from build123d import *

# Parameters (mm, degrees)
SKETCH1_W           = 150
SKETCH1_H           = 150
BOSS_EXTRUDE1_DEPTH = 1.5
CUT_EXTRUDE1_DEPTH  = 3
SKETCH3_R           = 1.55
CUT_EXTRUDE2_DEPTH  = 3
SKETCH6_R           = 1.3
SKETCH6_R_2         = 2.55
CUT_EXTRUDE9_DEPTH  = 3
SKETCH7_W           = 20
SKETCH7_H           = 50
SKETCH7_W_2         = 48
SKETCH7_H_2         = 40
SKETCH7_W_3         = 74
SKETCH7_H_3         = 46
CUT_EXTRUDE10_DEPTH = 3
FILLET1_R           = 4


with BuildPart() as part:
    # Sketch1 → Boss-Extrude1 (new body, symmetric)
    with BuildSketch(Plane(origin=(0, 0, 0), x_dir=(1, 0, 0), z_dir=(0, 1, 0))):
        Rectangle(SKETCH1_W, SKETCH1_H)
    extrude(amount=BOSS_EXTRUDE1_DEPTH, both=True)

    # Sketch2 → Cut-Extrude1 (cut)
    with BuildSketch(Plane(origin=(0, 1.5, 0), x_dir=(1, 0, 0), z_dir=(0, 1, 0))):
        Polygon((50.251262658, 75), (75, 75), (75, 50.251262658), align=None)
        Polygon((-75, 75), (-75, 50.251262658), (-50.251262658, 75), align=None)
        Polygon((-50.251262658, -75), (-75, -75), (-75, -50.251262658), align=None)
        Polygon((75, -75), (75, -50.251262658), (50.251262658, -75), align=None)
    extrude(amount=-CUT_EXTRUDE1_DEPTH, mode=Mode.SUBTRACT)

    # Sketch3 → Cut-Extrude2 (cut)
    with BuildSketch(Plane(origin=(0, 1.5, 0), x_dir=(1, 0, 0), z_dir=(0, 1, 0))):
        with Locations((69.343145751, 50.251262658)):
            Circle(SKETCH3_R)
        with Locations((50.251262658, 69.343145751)):
            Circle(SKETCH3_R)
        with Locations((-69.343145751, 50.251262658)):
            Circle(SKETCH3_R)
        with Locations((-50.251262658, 69.343145751)):
            Circle(SKETCH3_R)
        with Locations((-69.343145751, -50.251262658)):
            Circle(SKETCH3_R)
        with Locations((-50.251262658, -69.343145751)):
            Circle(SKETCH3_R)
        with Locations((69.343145751, -50.251262658)):
            Circle(SKETCH3_R)
        with Locations((50.251262658, -69.343145751)):
            Circle(SKETCH3_R)
    extrude(amount=-CUT_EXTRUDE2_DEPTH, mode=Mode.SUBTRACT)

    # Sketch6 → Cut-Extrude9 (cut)
    with BuildSketch(Plane(origin=(0, 1.5, 0), x_dir=(1, 0, 0), z_dir=(0, 1, 0))):
        with Locations((36.251262658, 16)):
            Circle(SKETCH6_R)
        with Locations((-21.748737342, 16)):
            Circle(SKETCH6_R)
        with Locations((36.251262658, 65)):
            Circle(SKETCH6_R)
        with Locations((-21.748737342, 65)):
            Circle(SKETCH6_R)
        with Locations((-44.656854249, 4)):
            Circle(SKETCH6_R_2)
        with Locations((-44.656854249, -53)):
            Circle(SKETCH6_R_2)
        with Locations((43.343145751, 4)):
            Circle(SKETCH6_R_2)
        with Locations((43.343145751, -53)):
            Circle(SKETCH6_R_2)
    extrude(amount=-CUT_EXTRUDE9_DEPTH, mode=Mode.SUBTRACT)

    # Sketch7 → Cut-Extrude10 (cut)
    with BuildSketch(Plane(origin=(0, 1.5, 0), x_dir=(1, 0, 0), z_dir=(0, 1, 0))):
        with Locations((61, 0)):
            Rectangle(SKETCH7_W, SKETCH7_H)
        with Locations((-61, 0)):
            Rectangle(SKETCH7_W, SKETCH7_H)
        with Locations((7.251262658, 40.5)):
            Rectangle(SKETCH7_W_2, SKETCH7_H_2)
        with Locations((-0.656854249, -24.5)):
            Rectangle(SKETCH7_W_3, SKETCH7_H_3)
    extrude(amount=-CUT_EXTRUDE10_DEPTH, mode=Mode.SUBTRACT)

    # Fillet1
    fillet1_edges = [part.edges().sort_by_distance(p)[0] for p in [
        (51, 0, 25),
        (51, 0, -25),
        (71, 0, -25),
        (71, 0, 25),
        (36.343145751, 0, 1.5),
        (36.343145751, 0, 47.5),
        (-37.656854249, 0, 47.5),
        (-37.656854249, 0, 1.5),
        (31.251262658, 0, -60.5),
        (31.251262658, 0, -20.5),
        (-16.748737342, 0, -20.5),
        (-16.748737342, 0, -60.5),
        (-71, 0, 25),
        (-71, 0, -25),
        (-51, 0, -25),
        (-51, 0, 25),
    ]]
    fillet(fillet1_edges, radius=FILLET1_R)


solid = part.part
Check sheet for the modelled part. Datum: model origin and axes. Units: mm. A direction names the side the tool comes from. Coordinates: 2 decimals unless noted, no trailing zeros. Loops run counter-clockwise (first coordinate to the right, second up) from the corner with the lowest first, then second, coordinate; pieces in that order, holes last. Notation, with made-up numbers: (32.25, -29.75) -> (60.25, -29.75) arc R24 ccw to (60.25, 9.25) -> close; hole circle Ø9 at (-27, 84). An arc over 180 degrees is marked (long way). Write item = value, one per line. Start each with the question number.
1. Depth check by flat-ended pin: P1, Ø3, axis at x = -50.25, z = 69.34, coming from the -Y side. Enter the tip coordinate at first touch or a pass-through.
2. Section check C-C on y = 0.3. Give the number of separate pieces and of enclosed holes in the cut face, then the cut area to 3 significant figures.
3. Section check D-D on z = 60. Record the cut outline in (x, y), then the cut area to 3 significant figures.
4. Tool access check on faces 4 (the cylindrical face through (-15.546, -0.021, -59.359)), 5 (the flat face through (-62.8, 0.02, -62.45)). Record the directions out of +Z, -Z, +X, -X, +Y, -Y that give a thin tool (end or side, any length) a straight path to the whole face; none if there is none.
5. Draft check along X on faces 1 (the cylindrical face through (40.796, 0.021, 52.888)), 2 (the flat face through (-62.8, 0.02, 62.45)), 3 (the flat face through (-1, -1.5, -1)). Enter one of: released by +X, released by -X, zero draft, split by the parting line, or undercut.
6. Section check B-B on z = -4. Record the cut outline in (x, y).
7. Material ranges on line 1 (Z direction, x = 43, y = 0.75); line 2 (X direction, y = -0.1, z = 6); line 3 (Z direction, x = 24, y = -1), recorded low to high.
8. Section check A-A on x = 15. Record the cut outline in (y, z).
Responses:
q1.P1 = through
q2.separate_pieces = 1
q2.enclosed_holes = 20
q2.area = 13,800 mm2
q3.outline = (-65.25, -1.5) -> (65.25, -1.5) -> (65.25, 1.5) -> (-65.25, 1.5) -> close
q3.area = 392 mm2
q4.face_4 = +Y, -Y
q4.face_5 = -Z, -X, +Y, -Y
q5.face_1 = undercut
q5.face_2 = released by -X
q5.face_3 = zero draft
q6.outline = (-75, -1.5) -> (-71, -1.5) -> (-71, 1.5) -> (-75, 1.5) -> close; (-51, -1.5) -> (-47.21, -1.5) -> (-47.21, 1.5) -> (-51, 1.5) -> close; (-42.11, -1.5) -> (40.79, -1.5) -> (40.79, 1.5) -> (-42.11, 1.5) -> close; (45.89, -1.5) -> (51, -1.5) -> (51, 1.5) -> (45.89, 1.5) -> close; (71, -1.5) -> (75, -1.5) -> (75, 1.5) -> (71, 1.5) -> close
q7.line_1 = -75 to -6.53, -1.47 to 50.47, 55.53 to 75
q7.line_2 = -75 to -71, -51 to -37.66, 36.34 to 51, 71 to 75
q7.line_3 = -75 to -60.5, -20.5 to 1.5, 47.5 to 75
q8.outline = (-1.5, -75) -> (1.5, -75) -> (1.5, -60.5) -> (-1.5, -60.5) -> close; (-1.5, -20.5) -> (1.5, -20.5) -> (1.5, 1.5) -> (-1.5, 1.5) -> close; (-1.5, 47.5) -> (1.5, 47.5) -> (1.5, 75) -> (-1.5, 75) -> close
